```python
from build123d import *

# Parameters (mm, degrees)
BOSS_EXTRUDE1_OUTLINE_R = 50
BOSS_EXTRUDE1_DEPTH     = 1.22
SKETCH2_R               = 1.025
CUT_EXTRUDE2_DEPTH      = 10


# Read off the part's stored shape, not the designer's step: Boss-Extrude1
with BuildPart() as part:
    # Boss-Extrude1 outline → Boss-Extrude1 (new body)
    with BuildSketch(Plane.XY):
        Circle(BOSS_EXTRUDE1_OUTLINE_R)
        with BuildLine():
            ThreePointArc((-10.640683383, -13.893374577), (-6.680080661, -16.174873179), (-2.263779528, -17.352962348))
            Line((-2.263779528, -17.352962348), (-1.802339331, -24.433615634))
            ThreePointArc((-1.802339331, -24.433615634), (-9.36241701, -22.64056421), (-15.980874836, -18.570450707))
            Line((-15.980874836, -18.570450707), (-10.640683383, -13.893374577))
        make_face(mode=Mode.SUBTRACT)
        with BuildLine():
            ThreePointArc((-17.348198754, -2.3), (-16.160892844, -6.713832175), (-13.871131205, -10.669663495))
            Line((-13.871131205, -10.669663495), (-18.551621667, -16.00272894))
            ThreePointArc((-18.551621667, -16.00272894), (-22.629525039, -9.389067926), (-24.431476591, -1.831106659))
            Line((-24.431476591, -1.831106659), (-17.348198754, -2.3))
        make_face(mode=Mode.SUBTRACT)
        with BuildLine():
            ThreePointArc((2.3, -17.348198754), (6.713832175, -16.160892844), (10.669663495, -13.871131205))
            Line((10.669663495, -13.871131205), (16.00272894, -18.551621667))
            ThreePointArc((16.00272894, -18.551621667), (9.389067926, -22.629525039), (1.831106659, -24.431476591))
            Line((1.831106659, -24.431476591), (2.3, -17.348198754))
        make_face(mode=Mode.SUBTRACT)
        with BuildLine():
            ThreePointArc((13.893374577, -10.640683383), (16.174873179, -6.680080661), (17.352962348, -2.263779528))
            Line((17.352962348, -2.263779528), (24.433615634, -1.802339331))
            ThreePointArc((24.433615634, -1.802339331), (22.64056421, -9.36241701), (18.570450707, -15.980874836))
            Line((18.570450707, -15.980874836), (13.893374577, -10.640683383))
        make_face(mode=Mode.SUBTRACT)
        with BuildLine():
            ThreePointArc((-13.893374577, 10.640683383), (-16.174873179, 6.680080661), (-17.352962348, 2.263779528))
            Line((-17.352962348, 2.263779528), (-24.433615634, 1.802339331))
            ThreePointArc((-24.433615634, 1.802339331), (-22.64056421, 9.36241701), (-18.570450707, 15.980874836))
            Line((-18.570450707, 15.980874836), (-13.893374577, 10.640683383))
        make_face(mode=Mode.SUBTRACT)
        with BuildLine():
            ThreePointArc((-2.3, 17.348198754), (-6.713832175, 16.160892844), (-10.669663495, 13.871131205))
            Line((-10.669663495, 13.871131205), (-16.00272894, 18.551621667))
            ThreePointArc((-16.00272894, 18.551621667), (-9.389067926, 22.629525039), (-1.831106659, 24.431476591))
            Line((-1.831106659, 24.431476591), (-2.3, 17.348198754))
        make_face(mode=Mode.SUBTRACT)
        with BuildLine():
            ThreePointArc((-1.5, -4.769696007), (-5, 0), (-1.5, 4.769696007))
            Line((-1.5, 4.769696007), (-1.5, 7))
            Line((-1.5, 7), (1.5, 7))
            Line((1.5, 7), (1.5, 4.769696007))
            ThreePointArc((1.5, 4.769696007), (5, 0), (1.5, -4.769696007))
            Line((1.5, -4.769696007), (1.5, -7))
            Line((1.5, -7), (-1.5, -7))
            Line((-1.5, -7), (-1.5, -4.769696007))
        make_face(mode=Mode.SUBTRACT)
        with BuildLine():
            ThreePointArc((17.348198754, 2.3), (16.160892844, 6.713832175), (13.871131205, 10.669663495))
            Line((13.871131205, 10.669663495), (18.551621667, 16.00272894))
            ThreePointArc((18.551621667, 16.00272894), (22.629525039, 9.389067926), (24.431476591, 1.831106659))
            Line((24.431476591, 1.831106659), (17.348198754, 2.3))
        make_face(mode=Mode.SUBTRACT)
        with BuildLine():
            ThreePointArc((10.640683383, 13.893374577), (6.680080661, 16.174873179), (2.263779528, 17.352962348))
            Line((2.263779528, 17.352962348), (1.802339331, 24.433615634))
            ThreePointArc((1.802339331, 24.433615634), (9.36241701, 22.64056421), (15.980874836, 18.570450707))
            Line((15.980874836, 18.570450707), (10.640683383, 13.893374577))
        make_face(mode=Mode.SUBTRACT)
    extrude(amount=BOSS_EXTRUDE1_DEPTH)

    # Sketch2 → Cut-Extrude2 (cut)
    with BuildSketch(Plane.XY):
        with Locations((0, 20)):
            Circle(SKETCH2_R)
        with Locations((14.142135624, 14.142135624)):
            Circle(SKETCH2_R)
        with Locations((20, 0)):
            Circle(SKETCH2_R)
        with Locations((14.142135624, -14.142135624)):
            Circle(SKETCH2_R)
        with Locations((0, -20)):
            Circle(SKETCH2_R)
        with Locations((-14.142135624, -14.142135624)):
            Circle(SKETCH2_R)
        with Locations((-20, 0)):
            Circle(SKETCH2_R)
        with Locations((-14.142135624, 14.142135624)):
            Circle(SKETCH2_R)
    extrude(amount=CUT_EXTRUDE2_DEPTH, mode=Mode.SUBTRACT)


solid = part.part
```
Check sheet for the modelled part. Datum: model origin and axes. Units: mm. Round coordinates to 2 decimals unless told otherwise and drop trailing zeros. Order: outer loops, then holes, each group sorted by start corner. A loop starts at its lowest first (then second) coordinate and runs counter-clockwise, first axis right, second up. Notation, with made-up numbers: (-13.5, -16.5) - (20.5, -16.5) arc R21 ccw to (20.5, 17.5) - close; hole circle Ø5 at (68, -19). An arc over 180 degrees is marked (long way). Answer as CSV lines item,"result". Start each with the question number.
1) Depth check by flat-ended pin: pin 1 (1.2 mm diameter, centred on x = 14.14, y = -14.14, fed in from +Z). Enter the tip coordinate at first touch or a pass-through.
2) Section check C-C (x = 30). Record the cut outline in (y, z), then the cut area to 3 significant figures.
3) Scan lines: probe 1 along X at (y, z) = (20, 0.95) (3 decimals); probe 2 along X at (y, z) = (-3, 0.3); probe 3 along Y at (x, z) = (18.5, 0.5). Record each from-to range of solid material in increasing order.
4) Section check A-A (x = 40). Record the cut outline in (y, z).
5) Draft check along X on faces 1 (the face through (16.185, 6.655, 0.601)), 2 (the face through (47.69, 15.02, 0.6)), 3 (the face through (-1, -10, 1.22)). Enter one of: +X half, -X half, draft (parallel to the pull), parting line (faces both ways), or undercut.
6) Section check B-B (z = 0.5). Give the number of separate pieces and of enclosed holes in the cut face, then the cut area to 3 significant figures.
Determined:
1,pin 1,"through"
2,outline,"(-40, 0) - (40, 0) - (40, 1.22) - (-40, 1.22) - close"
2,area,"97.6 mm^2"
3,probe 1,"-45.826 to -14.151, -2.124 to -1.025, 1.025 to 2.091, 14.151 to 45.826"
3,probe 2,"-49.91 to -24.32, -17.24 to -4, 4 to 17.24, 24.32 to 49.91"
3,probe 3,"-46.45 to -15.9, -2.19 to 2.22, 15.94 to 46.45"
4,outline,"(-30, 0) - (30, 0) - (30, 1.22) - (-30, 1.22) - close"
5,face 1,"undercut"
5,face 2,"parting line"
5,face 3,"draft"
6,separate pieces,"1"
6,enclosed holes,"17"
6,area,"7,040 mm^2"
